```python
from build123d import *

# Parameters (mm, degrees)
F0_W     = 50
F0_H     = 52.8824854079
F1_DEPTH = 50
F3_DEPTH = 50
F4_R     = 5
F5_DEPTH = 50.001
F6_W     = 17.3539984971
F6_H     = 12.1642492712
F7_DEPTH = 50.001


with BuildPart() as f1:
    # F0 (on Top) → F1 (new body)
    with BuildSketch(Plane.XY):
        with Locations((5.1456615329, 7.0626717061)):
            Rectangle(F0_W, F0_H)
    extrude(amount=F1_DEPTH)

    # F2 (on face) → F3 (cut)
    with BuildSketch(Plane.YZ.offset(30.1456615329)):
        Polygon((-19.3785709979, 50), (-19.3785709979, 36.2214259803), (0, 50), align=None)
    extrude(amount=-F3_DEPTH, mode=Mode.SUBTRACT)

    # F4 (on face) → F5 (cut, through all)
    with BuildSketch(Plane.YZ.offset(30.1456615329)):
        with Locations((-12.5574155126, 6.8796549415)):
            Circle(F4_R)
        with Locations((25.9205371111, 43.0046210508)):
            Circle(F4_R)
    extrude(amount=-F5_DEPTH, mode=Mode.SUBTRACT)

    # F6 (on face) → F7 (cut, through all)
    with BuildSketch(Plane.YZ.offset(30.1456615329)):
        Polygon((33.50391441, 0), (33.50391441, 25), (14.1253471375, 25), (14.1253471375, 10.190429166), align=None)
        with Locations((8.6769992486, 43.9178753644)):
            Rectangle(F6_W, F6_H)
    extrude(amount=-F7_DEPTH, mode=Mode.SUBTRACT)


solid = f1.part
```
Part model, mm, in its own coordinate system. A direction names the side the tool comes from. Round coordinates to 2 decimals unless told otherwise and drop trailing zeros. Loops run counter-clockwise (first coordinate to the right, second up) from the corner with the lowest first, then second, coordinate; pieces in that order, holes last. Notation, with made-up numbers: (61, 17) -> (82, 17) arc R19 ccw to (82, 32) -> close; hole circle Ø3 at (56, 62.5). An arc over 180 degrees is marked (long way). Use CSV: the item, a comma, the result in double quotes. Start each with the question number.
1) Cut at A-A, the plane y = 28. Write the cut outline in (x, z), plus the area to 3 significant figures.
2) Drop flat-ended pins along their axis: P1, Ø8.5, axis at x = -1.5, y = 7.5, coming from the +Z side; P2, Ø6, axis at x = 12.5, y = 24, coming from the -Z side; P3, Ø2, axis at x = 22, y = -2.5, coming from the +Z side; P4, Ø13.5, axis at x = 9.5, z = 43.5, coming from the -Y side. Give the stop position or say it passes through.
3) Cut at D-D, the plane x = -11. Write the cut outline in (y, z).
4) Which spindle directions (+Z, -Z, +X, -X, +Y, -Y) get a long thin tool onto all of the face, cutting with end or side? Do faces 1 (the flat face through (5.496, 23.679, 5.167)), 2 (the flat face through (5, -19.379, 18)), 3 (the flat face through (5, 17.354, 44)). Say none if no direction does.
5) Cut at B-B, the plane z = 44.5. Write the cut outline in (x, y), plus the area to 3 significant figures.
6) Pull direction Y, two halves, no side cores. Call faces 4 (the flat face through (5.496, -9.825, 43.014)), 5 (the flat face through (-19.854, 1, 25)), 6 (the cylindrical face through (5.496, 24.837, 38.124)): +Y half, -Y half, draft (parallel to the pull), parting line (faces both ways), or undercut.
7) Wall check: L1, parallel to Y at x = 8, z = 42.5 (3 decimals); L2, parallel to Z at x = -11.5, y = 26.5; L3, parallel to Z at x = 13, y = 10. Give the ranges that are in metal, low to high. Write a range as [from, to].
8) Cut at C-C, the plane y = -14. Write the cut outline in (x, z), plus the area to 3 significant figures.
Determined:
1,outline,"(-19.85, 0) -> (30.15, 0) -> (30.15, 2.89) -> (-19.85, 2.89) -> close; (-19.85, 25) -> (30.15, 25) -> (30.15, 38.46) -> (-19.85, 38.46) -> close; (-19.85, 47.55) -> (30.15, 47.55) -> (30.15, 50) -> (-19.85, 50) -> close"
1,area,"940 mm2"
2,P1,"stops at z = 37.84"
2,P2,"stops at z = 0"
2,P3,"stops at z = 48.93"
2,P4,"stops at y = -18.64"
3,outline,"(-19.38, 0) -> (33.5, 0) -> (14.13, 10.19) -> (14.13, 25) -> (33.5, 25) -> (33.5, 50) -> (17.35, 50) -> (17.35, 37.84) -> (0, 37.84) -> (0, 50) -> (-19.38, 36.22) -> close; hole circle Ø10 at (-12.56, 6.88); hole circle Ø10 at (25.92, 43)"
4,face 1,"+X, -X, +Y"
4,face 2,"+Z, -Z, +X, -X, -Y"
4,face 3,"+Z, +X, -X"
5,outline,"(-19.85, -7.74) -> (30.15, -7.74) -> (30.15, 0) -> (-19.85, 0) -> close; (-19.85, 17.35) -> (30.15, 17.35) -> (30.15, 21.15) -> (-19.85, 21.15) -> close; (-19.85, 30.69) -> (30.15, 30.69) -> (30.15, 33.5) -> (-19.85, 33.5) -> close"
5,area,"717 mm2"
6,face 4,"-Y half"
6,face 5,"draft"
6,face 6,"undercut"
7,L1,"y = [-10.548, 0], [17.354, 20.946], [30.895, 33.504]"
7,L2,"z = [0, 3.68], [25, 38.04], [47.97, 50]"
7,L3,"z = [0, 37.84]"
8,outline,"(-19.85, 0) -> (30.15, 0) -> (30.15, 2.09) -> (-19.85, 2.09) -> close; (-19.85, 11.67) -> (30.15, 11.67) -> (30.15, 40.05) -> (-19.85, 40.05) -> close"
8,area,"1,520 mm2"
